Input: dimensioned drawing with shaded views. Units: mm. Origin: part minimum x, y, z. Give positions to 0.01 mm unless a question says otherwise; leave off trailing zeros. Write each loop counter-clockwise with the first axis right and the second up, starting at its lowest first coordinate (ties: lowest second). Pieces come first, ordered by that corner, then holes.
Q1. Section C-C (x = 25). Return the cut outline in (y, z), plus the area to 3 significant figures.
Q2. Pin query (flat end, axial travel): pin 1 Ø1 at (y, z) = (3, 6.5) entering from -X; pin 2 Ø6.5 at (x, z) = (22.5, 20) entering from -Y; pin 3 Ø3 at (x, z) = (40.5, 9.5) entering from -Y; pin 4 Ø3 at (x, z) = (40, 42) entering from -Y. Return the tip coordinate at first contact, or that it passes through.
Q3. Section A-A (z = 9.5). Return the cut outline in (x, y).
Q4. Section B-B (y = 5). Return the cut outline in (x, z).
Q5. Mould query, pull axis Z, two halves, no side actions, for the marked faces 1, 2 and 3. Classes: +Z half, -Z half, draft (parallel to the pull), parting line (faces both ways), or undercut.
Q6. Section D-D (x = 40.5). Return the cut outline in (y, z), plus the area to 3 significant figures.
Q7. Line query: line 1 (Z direction, x = 9.5, y = 5.9); line 2 (Z direction, x = 25, y = 3.8); line 3 (X direction, y = 0.75, z = 43.5). Output: solid intervals per line, ascending.
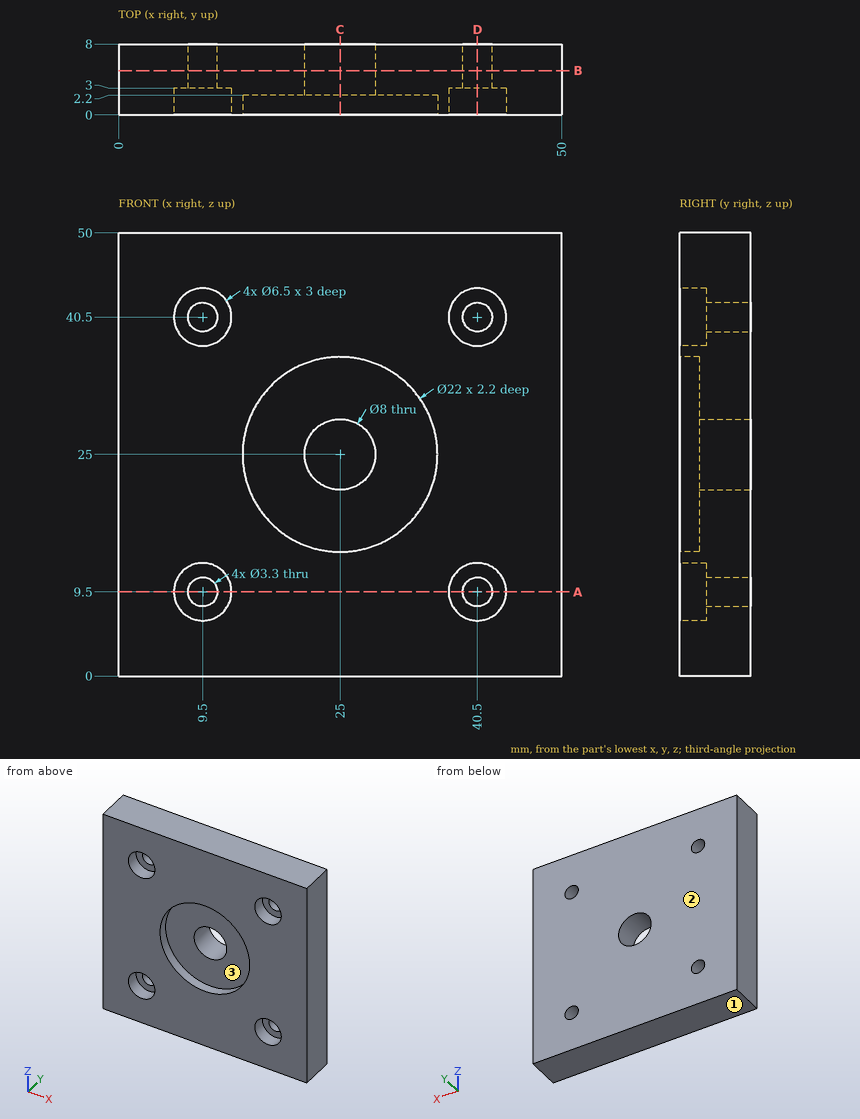
Computed:
1. outline: (0, 0) - (8, 0) - (8, 21) - (2.2, 21) - (2.2, 14) - (0, 14) - close; (0, 36) - (2.2, 36) - (2.2, 29) - (8, 29) - (8, 50) - (0, 50) - close
1. area: 305 mm2
2. pin 1: stops at x = 0
2. pin 2: stops at y = 2.2
2. pin 3: passes through
2. pin 4: stops at y = 3
3. outline: (0, 0) - (6.25, 0) - (6.25, 3) - (7.85, 3) - (7.85, 8) - (0, 8) - close; (11.15, 3) - (12.75, 3) - (12.75, 0) - (37.25, 0) - (37.25, 3) - (38.85, 3) - (38.85, 8) - (11.15, 8) - close; (42.15, 3) - (43.75, 3) - (43.75, 0) - (50, 0) - (50, 8) - (42.15, 8) - close
4. outline: (0, 0) - (50, 0) - (50, 50) - (0, 50) - close; hole circle Ø3.3 at (9.5, 9.5); hole circle Ø3.3 at (9.5, 40.5); hole circle Ø8 at (25, 25); hole circle Ø3.3 at (40.5, 9.5); hole circle Ø3.3 at (40.5, 40.5)
5. face 1: -Z half
5. face 2: draft
5. face 3: undercut
6. outline: (0, 0) - (8, 0) - (8, 7.85) - (3, 7.85) - (3, 6.25) - (0, 6.25) - close; (0, 12.75) - (3, 12.75) - (3, 11.15) - (8, 11.15) - (8, 38.85) - (3, 38.85) - (3, 37.25) - (0, 37.25) - close; (0, 43.75) - (3, 43.75) - (3, 42.15) - (8, 42.15) - (8, 50) - (0, 50) - close
6. area: 328 mm2
7. line 1: z = 0 to 7.85, 11.15 to 38.85, 42.15 to 50
7. line 2: z = 0 to 21, 29 to 50
7. line 3: x = 0 to 8.25, 10.75 to 39.25, 41.75 to 50
